```python
from build123d import *

# Parameters (mm, degrees)
SKETCH1_W                      = 152.4
SKETCH1_H                      = 101.6
BASE_FLANGE1_DEPTH             = 1.29032
EDGE_FLANGE1_STRIP_W           = 8.97128
EDGE_FLANGE1_STRIP_H           = 1.29032
EDGE_FLANGE1_STRIP_CUT_DEPTH   = 152.4
EDGE_FLANGE1_STRIP_2_W         = 8.97128
EDGE_FLANGE1_STRIP_2_H         = 1.29032
EDGE_FLANGE1_STRIP_CUT_2_DEPTH = 152.4
EDGE_FLANGE1_DEPTH             = 152.4
EDGE_FLANGE1_BEND_DEPTH        = 152.4
EDGE_FLANGE2_DEPTH             = 95.20936
EDGE_FLANGE2_BEND_DEPTH        = 95.20936
SKETCH22_R                     = 19.249999981
SKETCH22_R_2                   = 1
CUT_EXTRUDE1_DEPTH             = 2.54
CUT_EXTRUDE2_REACH             = 141.067
SKETCH23_R                     = 3.81


# Sheet-metal steps are written as plain solids
with BuildPart() as part:
    # Sketch1 → Base-Flange1 (new body)
    with BuildSketch(Plane(origin=(0, 0, 0), x_dir=(1, 0, 0), z_dir=(0, 1, 0))):
        Rectangle(SKETCH1_W, SKETCH1_H)
    extrude(amount=-BASE_FLANGE1_DEPTH)

    # Edge-Flange1 strip (across the edge) → Edge-Flange1 strip cut (cut)
    with BuildSketch(Plane(origin=(76.2, -1.29032, 50.8), x_dir=(0, 0, -1), z_dir=(-1, 0, 0))):
        with Locations((-1.29032, -0.64516)):
            Rectangle(EDGE_FLANGE1_STRIP_W, EDGE_FLANGE1_STRIP_H)
    extrude(amount=EDGE_FLANGE1_STRIP_CUT_DEPTH, mode=Mode.SUBTRACT)

    # Edge-Flange1 strip 2 (across the edge) → Edge-Flange1 strip cut 2 (cut)
    with BuildSketch(Plane(origin=(-76.2, -1.29032, -50.8), x_dir=(0, 0, 1), z_dir=(1, 0, 0))):
        with Locations((-1.29032, -0.64516)):
            Rectangle(EDGE_FLANGE1_STRIP_2_W, EDGE_FLANGE1_STRIP_2_H)
    extrude(amount=EDGE_FLANGE1_STRIP_CUT_2_DEPTH, mode=Mode.SUBTRACT)

    # Edge-Flange1 section (across the edge) → Edge-Flange1 (add)
    with BuildSketch(Plane(origin=(76.2, -1.29032, 50.8), x_dir=(0, 0, -1), z_dir=(-1, 0, 0))):
        with BuildLine():
            Line((0, 1.905), (0, 50.8))
            Line((0, 50.8), (1.29032, 50.8))
            Line((1.29032, 50.8), (1.29032, 1.905))
            ThreePointArc((1.29032, 1.905), (1.848281582, 0.557961582), (3.19532, 0))
            Line((3.19532, 0), (3.19532, -1.29032))
            ThreePointArc((3.19532, -1.29032), (0.93588756, -0.35443244), (0, 1.905))
        make_face()
    extrude(amount=EDGE_FLANGE1_DEPTH)

    # Edge-Flange1 section 2 (across the edge) → Edge-Flange1 bend (add)
    with BuildSketch(Plane(origin=(-76.2, -1.29032, -50.8), x_dir=(0, 0, 1), z_dir=(1, 0, 0))):
        with BuildLine():
            Line((0, 1.905), (0, 50.8))
            Line((0, 50.8), (1.29032, 50.8))
            Line((1.29032, 50.8), (1.29032, 1.905))
            ThreePointArc((1.29032, 1.905), (1.848281582, 0.557961582), (3.19532, 0))
            Line((3.19532, 0), (3.19532, -1.29032))
            ThreePointArc((3.19532, -1.29032), (0.93588756, -0.35443244), (0, 1.905))
        make_face()
    extrude(amount=EDGE_FLANGE1_BEND_DEPTH)

    # Edge-Flange2 section (across the edge) → Edge-Flange2 (add)
    with BuildSketch(Plane(origin=(-78.105, -1.29032, 47.60468), x_dir=(1, 0, 0), z_dir=(0, 0, -1))):
        with BuildLine():
            Line((-1.29032, 1.905), (-1.29032, 12.7))
            Line((-1.29032, 12.7), (0, 12.7))
            Line((0, 12.7), (0, 1.905))
            ThreePointArc((0, 1.905), (0.557961582, 0.557961582), (1.905, 0))
            Line((1.905, 0), (1.905, -1.29032))
            ThreePointArc((1.905, -1.29032), (-0.35443244, -0.35443244), (-1.29032, 1.905))
        make_face()
    extrude(amount=EDGE_FLANGE2_DEPTH)

    # Edge-Flange2 section 2 (across the edge) → Edge-Flange2 bend (add)
    with BuildSketch(Plane(origin=(78.105, -1.29032, -47.60468), x_dir=(-1, 0, 0), z_dir=(0, 0, 1))):
        with BuildLine():
            Line((-1.29032, 1.905), (-1.29032, 12.7))
            Line((-1.29032, 12.7), (0, 12.7))
            Line((0, 12.7), (0, 1.905))
            ThreePointArc((0, 1.905), (0.557961582, 0.557961582), (1.905, 0))
            Line((1.905, 0), (1.905, -1.29032))
            ThreePointArc((1.905, -1.29032), (-0.35443244, -0.35443244), (-1.29032, 1.905))
        make_face()
    extrude(amount=EDGE_FLANGE2_BEND_DEPTH)

    # Sketch22 → Cut-Extrude1 (cut)
    with BuildSketch(Plane(origin=(0, 0, 0), x_dir=(1, 0, 0), z_dir=(0, 1, 0))):
        with Locations(Location((34.925, 19.05, 0), (0, 0, 270))):
            Circle(SKETCH22_R)
        with Locations(Location((19.925, 34.8, 0), (0, 0, 270))):
            Circle(SKETCH22_R_2)
        with Locations(Location((49.925, 34.8, 0), (0, 0, 270))):
            Circle(SKETCH22_R_2)
        with Locations(Location((49.925, 3.3, 0), (0, 0, 270))):
            Circle(SKETCH22_R_2)
        with Locations(Location((19.925, 3.3, 0), (0, 0, 270))):
            Circle(SKETCH22_R_2)
        with Locations(Location((-19.925, 3.3, 0), (0, 0, 90))):
            Circle(SKETCH22_R_2)
        with Locations(Location((-49.925, 3.3, 0), (0, 0, 90))):
            Circle(SKETCH22_R_2)
        with Locations(Location((-49.925, 34.8, 0), (0, 0, 90))):
            Circle(SKETCH22_R_2)
        with Locations(Location((-19.925, 34.8, 0), (0, 0, 90))):
            Circle(SKETCH22_R_2)
        with Locations(Location((-34.925, 19.05, 0), (0, 0, 90))):
            Circle(SKETCH22_R)
    extrude(amount=-CUT_EXTRUDE1_DEPTH, mode=Mode.SUBTRACT)

    # Sketch23 → Cut-Extrude2 (cut, up to next)
    with BuildSketch(Plane(origin=(0, 0, -50.8), x_dir=(-1, 0, 0), z_dir=(0, 0, -1)), mode=Mode.PRIVATE) as cut_extrude2_sk1:
        with Locations(Location((60.325, -25.4, 0), (0, 0, 90))):
            Circle(SKETCH23_R)
    cut_extrude2_tool1 = extrude(cut_extrude2_sk1.sketch, amount=-CUT_EXTRUDE2_REACH, mode=Mode.PRIVATE) & part.part
    # Sketch23 → Cut-Extrude2 (cut, up to next)
    with BuildSketch(Plane(origin=(0, 0, -50.8), x_dir=(-1, 0, 0), z_dir=(0, 0, -1)), mode=Mode.PRIVATE) as cut_extrude2_sk2:
        with Locations(Location((-60.325, -25.4, 0), (0, 0, 90))):
            Circle(SKETCH23_R)
    cut_extrude2_tool2 = extrude(cut_extrude2_sk2.sketch, amount=-CUT_EXTRUDE2_REACH, mode=Mode.PRIVATE) & part.part
    add(cut_extrude2_tool1.solids().sort_by_distance((-60.325, -25.4, -50.8))[0], mode=Mode.SUBTRACT)
    add(cut_extrude2_tool2.solids().sort_by_distance((60.325, -25.4, -50.8))[0], mode=Mode.SUBTRACT)


solid = part.part
```
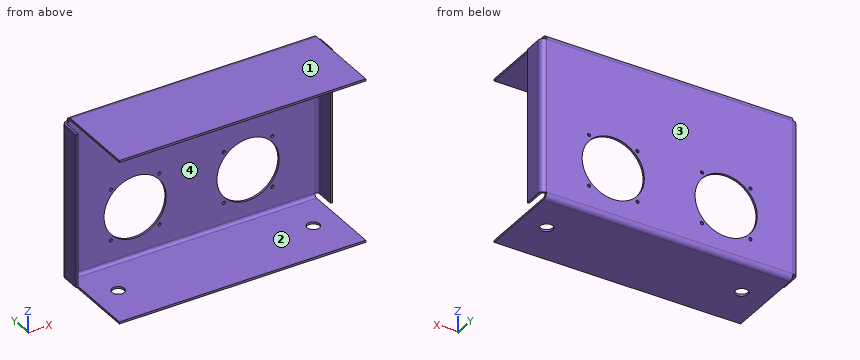
Could you check a few things on this model? Use its own coordinates, in mm. Face numbers are marked on the shaded views. A direction names the side the tool comes from. Coordinates: 2 decimals unless noted, no trailing zeros. Write each loop counter-clockwise with the first axis right and the second up, starting at its lowest first coordinate (ties: lowest second). Pieces come first, ordered by that corner, then holes. Notation, with made-up numbers: (-7.75, 24.5) - (-1.75, 24.5) arc R22 ccw to (-1.75, 45.5) - close; hole circle Ø1 at (23.5, 64). An arc over 180 degrees is marked (long way). Use a Markdown table: item, result.
Q1. Imagine slicing it at A-A (y = -44). List the corners of the cut face in (x, z) for me, and give its area (3 significant figures).
Geometry check:
| item | result |
|---|---|
| outline | (-76.2, -50.8) - (76.2, -50.8) - (76.2, -49.51) - (-76.2, -49.51) - close; (-76.2, 49.51) - (76.2, 49.51) - (76.2, 50.8) - (-76.2, 50.8) - close |
| area | 393 mm2 |
Q2. Imagine slicing it at C-C (y = -25.4). List the corners of the cut face in (x, z) for me (3 decimals), and give its area (3 significant figures).
Geometry check:
| item | result |
|---|---|
| outline | (-76.2, -50.8) - (-64.135, -50.8) - (-64.135, -49.51) - (-76.2, -49.51) - close; (-76.2, 49.51) - (76.2, 49.51) - (76.2, 50.8) - (-76.2, 50.8) - close; (-56.515, -50.8) - (56.515, -50.8) - (56.515, -49.51) - (-56.515, -49.51) - close; (64.135, -50.8) - (76.2, -50.8) - (76.2, -49.51) - (64.135, -49.51) - close |
| area | 374 mm2 |
Q3. Imagine slicing it at B-B (z = -19.05). List the corners of the cut face in (x, y) for me (3 decimals), and give its area (3 significant figures).
Geometry check:
| item | result |
|---|---|
| outline | (-79.395, -13.99) - (-78.105, -13.99) - (-78.105, -3.195) arc R1.905 cw to (-76.2, -1.29) - (-54.175, -1.29) - (-54.175, 0) - (-76.2, 0) arc R3.195 ccw to (-79.395, -3.195) - close; (-15.675, -1.29) - (15.675, -1.29) - (15.675, 0) - (-15.675, 0) - close; (54.175, -1.29) - (76.2, -1.29) arc R1.905 cw to (78.105, -3.195) - (78.105, -13.99) - (79.395, -13.99) - (79.395, -3.195) arc R3.195 ccw to (76.2, 0) - (54.175, 0) - close |
| area | 135 mm2 |
Q4. I'm going to push flat-ended pins straight in: pin 1 Ø1.6 at (y, z) = (-21.5, 48.5) entering from +X; pin 2 Ø1 at (x, z) = (78.5, 1) entering from -Y; pin 3 Ø2.5 at (y, z) = (-32, 49.5) entering from -X; pin 4 Ø7 at (x, y) = (60.325, -25.4) entering from -Z. Where does each tip first touch, or does it pass through?
Geometry check:
| item | result |
|---|---|
| pin 1 | passes through |
| pin 2 | stops at y = -13.99 |
| pin 3 | stops at x = -76.2 |
| pin 4 | stops at z = 49.51 |
Q5. Please list where these lines run through material, in increasing order: L1, parallel to Z at x = 60, y = -10.5; L2, parallel to Y at x = -19, z = 40; L3, parallel to X at y = -9, z = -31 (3 decimals).
Geometry check:
| item | result |
|---|---|
| L1 | z = -50.8 to -49.51, 49.51 to 50.8 |
| L2 | y = -1.29 to 0 |
| L3 | x = -79.395 to -78.105, 78.105 to 79.395 |
Q6. Imagine slicing it at D-D (z = -41). List the corners of the cut face in (x, y) for me (3 decimals), and give its area (3 significant figures).
Geometry check:
| item | result |
|---|---|
| outline | (-79.395, -13.99) - (-78.105, -13.99) - (-78.105, -3.195) arc R1.905 cw to (-76.2, -1.29) - (76.2, -1.29) arc R1.905 cw to (78.105, -3.195) - (78.105, -13.99) - (79.395, -13.99) - (79.395, -3.195) arc R3.195 ccw to (76.2, 0) - (-76.2, 0) arc R3.195 ccw to (-79.395, -3.195) - close |
| area | 235 mm2 |
Q7. Thinking about a two-plate mould opening in X: for the marked faces 3 and 4, which applies, +X half, -X half, draft (parallel to the pull), parting line (faces both ways), or undercut?
Geometry check:
| item | result |
|---|---|
| face 3 | draft |
| face 4 | undercut |
Q8. Which directions (+Z, -Z, +X, -X, +Y, -Y) give clear straight access to the entire face, cutting with the end or side of a thin tool? Please do the marked faces 1 and 2.
Geometry check:
| item | result |
|---|---|
| face 1 | +Z, +X, -X, +Y, -Y |
| face 2 | +X, -X, -Y |
